from build123d import *

# Parameters (mm, degrees)
F0_R     = 10.925
F1_DEPTH = 8


with BuildPart() as f1:
    # F0 (on Front) → F1 (new body)
    with BuildSketch(Plane.XZ):
        Polygon((137.5925300597, 43.0939033628), (138.203267445, 43.0939033628), (132.6625055075, 50.7201079193), (132.6625055075, 44.6957654427), align=None)
        Polygon((132.6625055075, 66.4920412828), (138.3919956762, 68.353665488), (141.9330153387, 73.2274609315), (132.6625055075, 76.2396321698), align=None)
        with BuildLine():
            Line((152.4504447694, 74.5233945768), (153.3919956762, 73.2274609315))
            Line((153.3919956762, 73.2274609315), (162.6625055075, 76.2396321698))
            Line((162.6625055075, 76.2396321698), (162.6625055075, 93.0939033628))
            ThreePointArc((162.6625055075, 93.0939033628), (161.1980394134, 96.6294372687), (157.6625055075, 98.0939033628))
            Line((157.6625055075, 98.0939033628), (137.6625055075, 98.0939033628))
            ThreePointArc((137.6625055075, 98.0939033628), (134.1269716015, 96.6294372687), (132.6625055075, 93.0939033628))
            Line((132.6625055075, 93.0939033628), (132.6625055075, 76.2396321698))
            Line((132.6625055075, 76.2396321698), (141.9330153387, 73.2274609315))
            Line((141.9330153387, 73.2274609315), (142.8745662455, 74.5233945768))
            Line((142.8745662455, 74.5233945768), (146.8630398909, 71.6255988516))
            Line((146.8630398909, 71.6255988516), (147.6625055075, 71.3658367263))
            Line((147.6625055075, 71.3658367263), (148.461971124, 71.6255988516))
            Line((148.461971124, 71.6255988516), (152.4504447694, 74.5233945768))
        make_face()
        with Locations((147.6625055075, 85.5939033628)):
            Circle(F0_R, mode=Mode.SUBTRACT)
        Polygon((153.3919956762, 73.2274609315), (156.9330153387, 68.353665488), (162.6625055075, 66.4920412828), (162.6625055075, 76.2396321698), align=None)
        Polygon((147.9678742002, 71.2666164235), (156.9330153387, 68.353665488), (153.3919956762, 73.2274609315), (148.461971124, 71.6255988516), align=None)
        Polygon((138.5807239074, 43.0939033628), (156.7442871075, 43.0939033628), (162.3571368148, 60.3684785034), (147.6625055075, 71.0447530815), (132.9678742002, 60.3684785034), align=None)
        with Locations((147.6625055075, 55.5939033628)):
            Circle(F0_R, mode=Mode.SUBTRACT)
        Polygon((147.6625055075, 30.0743791122), (153.3919956762, 37.960345794), (147.6625055075, 39.8219699992), (141.9330153387, 37.960345794), align=None)
        with BuildLine():
            Line((137.7558134621, 16.4389872893), (147.6625055075, 30.0743791122))
            Line((147.6625055075, 30.0743791122), (141.9330153387, 37.960345794))
            Line((141.9330153387, 37.960345794), (140.4095539694, 37.4653431886))
            Line((140.4095539694, 37.4653431886), (138.8860926001, 42.1540751645))
            Line((138.8860926001, 42.1540751645), (138.3919956762, 42.8341412375))
            Line((138.3919956762, 42.8341412375), (137.5925300597, 43.0939033628))
            Line((137.5925300597, 43.0939033628), (132.6625055075, 43.0939033628))
            Line((132.6625055075, 43.0939033628), (132.6625055075, 44.6957654427))
            Line((132.6625055075, 44.6957654427), (123.3919956762, 47.707936681))
            Line((123.3919956762, 47.707936681), (113.4853036309, 34.0725448581))
            ThreePointArc((113.4853036309, 34.0725448581), (112.5919468998, 30.3514462714), (114.5914623413, 27.0885336247))
            Line((114.5914623413, 27.0885336247), (130.7718022288, 15.3328285789))
            ThreePointArc((130.7718022288, 15.3328285789), (134.4929008155, 14.4394718478), (137.7558134621, 16.4389872893))
        make_face()
        with Locations((130.0289479387, 31.3233935315)):
            Circle(F0_R, mode=Mode.SUBTRACT)
        with BuildLine():
            Line((162.6625055075, 44.6957654427), (162.6625055075, 43.0939033628))
            Line((162.6625055075, 43.0939033628), (157.7324809553, 43.0939033628))
            Line((157.7324809553, 43.0939033628), (156.9330153387, 42.8341412375))
            Line((156.9330153387, 42.8341412375), (156.4389184148, 42.1540751645))
            Line((156.4389184148, 42.1540751645), (154.9154570455, 37.4653431886))
            Line((154.9154570455, 37.4653431886), (153.3919956762, 37.960345794))
            Line((153.3919956762, 37.960345794), (147.6625055075, 30.0743791122))
            Line((147.6625055075, 30.0743791122), (157.5691975528, 16.4389872893))
            ThreePointArc((157.5691975528, 16.4389872893), (160.8321101995, 14.4394718478), (164.5532087862, 15.3328285789))
            Line((164.5532087861, 15.3328285789), (180.7335486736, 27.0885336247))
            ThreePointArc((180.7335486736, 27.0885336247), (182.7330641152, 30.3514462714), (181.8397073841, 34.0725448581))
            Line((181.8397073841, 34.0725448581), (171.9330153387, 47.707936681))
            Line((171.9330153387, 47.707936681), (162.6625055075, 44.6957654427))
        make_face()
        with Locations((165.2960630762, 31.3233935315)):
            Circle(F0_R, mode=Mode.SUBTRACT)
        with BuildLine():
            Line((166.20352517, 55.5939033628), (171.9330153387, 47.707936681))
            Line((171.9330153387, 47.707936681), (187.9623797842, 52.9161929074))
            ThreePointArc((187.9623797842, 52.9161929074), (190.8723274332, 55.4015229902), (191.1725773938, 59.2165604607))
            Line((191.1725773938, 59.2165604607), (184.9922375063, 78.2376907866))
            ThreePointArc((184.9922375063, 78.2376907866), (182.5069074235, 81.1476384357), (178.6918699529, 81.4478883962))
            Line((178.6918699529, 81.4478883962), (162.6625055075, 76.2396321698))
            Line((162.6625055075, 76.2396321698), (162.6625055075, 66.4920412828))
            Line((162.6625055075, 66.4920412828), (164.1859668768, 65.9970386775))
            Line((164.1859668768, 65.9970386775), (162.6625055075, 61.3083067016))
            Line((162.6625055075, 61.3083067016), (162.6625055075, 60.4676988062))
            Line((162.6625055075, 60.4676988062), (163.1566024313, 59.7876327333))
            Line((163.1566024313, 59.7876327333), (167.1450760767, 56.8898370081))
            Line((167.1450760767, 56.8898370081), (166.20352517, 55.5939033628))
        make_face()
        with Locations((176.1942009963, 64.864413194)):
            Circle(F0_R, mode=Mode.SUBTRACT)
        Polygon((162.6625055075, 50.7201079193), (162.6625055075, 44.6957654427), (171.9330153387, 47.707936681), (166.20352517, 55.5939033628), align=None)
        Polygon((162.6625055075, 60.1466151614), (162.6625055075, 50.7201079193), (166.20352517, 55.5939033628), (163.1566024313, 59.7876327333), align=None)
        Polygon((163.1566024313, 59.7876327333), (166.20352517, 55.5939033628), (167.1450760767, 56.8898370081), align=None)
        Polygon((156.7442871075, 43.0939033628), (157.1217435699, 43.0939033628), (162.6625055075, 50.7201079193), (162.6625055075, 60.1466151614), (162.3571368148, 60.3684785034), align=None)
        Polygon((157.1217435699, 43.0939033628), (157.7324809553, 43.0939033628), (162.6625055075, 44.6957654427), (162.6625055075, 50.7201079193), align=None)
        Polygon((157.7324809553, 43.0939033628), (162.6625055075, 43.0939033628), (162.6625055075, 44.6957654427), align=None)
        Polygon((154.9154570455, 37.4653431886), (156.4389184148, 42.1540751645), (153.3919956762, 37.960345794), align=None)
        Polygon((153.3919956762, 37.960345794), (156.4389184148, 42.1540751645), (156.627646646, 42.7349209346), (147.6625055075, 39.8219699992), align=None)
        Polygon((156.627646646, 42.7349209346), (156.7442871075, 43.0939033628), (138.5807239074, 43.0939033628), (138.6973643689, 42.7349209346), (147.6625055075, 39.8219699992), align=None)
        Polygon((141.9330153387, 37.960345794), (147.6625055075, 39.8219699992), (138.6973643689, 42.7349209346), (138.8860926001, 42.1540751645), align=None)
        Polygon((140.4095539694, 37.4653431886), (141.9330153387, 37.960345794), (138.8860926001, 42.1540751645), align=None)
        Polygon((138.203267445, 43.0939033628), (138.5807239074, 43.0939033628), (132.9678742002, 60.3684785034), (132.6625055075, 60.1466151614), (132.6625055075, 50.7201079193), align=None)
        Polygon((132.6625055075, 43.0939033628), (137.5925300597, 43.0939033628), (132.6625055075, 44.6957654427), align=None)
        Polygon((132.6625055075, 44.6957654427), (132.6625055075, 50.7201079193), (129.121485845, 55.5939033628), (123.3919956762, 47.707936681), align=None)
        Polygon((129.121485845, 55.5939033628), (132.6625055075, 50.7201079193), (132.6625055075, 60.1466151614), (132.1684085836, 59.7876327333), align=None)
        Polygon((128.1799349382, 56.8898370081), (129.121485845, 55.5939033628), (132.1684085836, 59.7876327333), align=None)
        Polygon((132.6625055075, 61.3083067016), (132.8512337387, 60.7274609315), (138.3919956762, 68.353665488), (132.6625055075, 66.4920412828), align=None)
        Polygon((131.1390441382, 65.9970386775), (132.6625055075, 61.3083067016), (132.6625055075, 66.4920412828), align=None)
        Polygon((132.8512337387, 60.7274609315), (132.9678742002, 60.3684785034), (147.6625055075, 71.0447530815), (147.3571368148, 71.2666164235), (138.3919956762, 68.353665488), align=None)
        Polygon((141.9330153387, 73.2274609315), (146.8630398909, 71.6255988516), (142.8745662455, 74.5233945768), align=None)
        Polygon((138.3919956762, 68.353665488), (147.3571368148, 71.2666164235), (146.8630398909, 71.6255988516), (141.9330153387, 73.2274609315), align=None)
        Polygon((147.6625055075, 71.0447530815), (162.3571368148, 60.3684785034), (162.4737772763, 60.7274609315), (156.9330153387, 68.353665488), (147.9678742002, 71.2666164235), align=None)
        Polygon((156.9330153387, 68.353665488), (162.4737772763, 60.7274609315), (162.6625055075, 61.3083067016), (162.6625055075, 66.4920412828), align=None)
        Polygon((162.6625055075, 66.4920412828), (162.6625055075, 61.3083067016), (164.1859668768, 65.9970386775), align=None)
        Polygon((148.461971124, 71.6255988516), (153.3919956762, 73.2274609315), (152.4504447694, 74.5233945768), align=None)
        with BuildLine():
            Line((123.3919956762, 47.707936681), (129.121485845, 55.5939033628))
            Line((129.121485845, 55.5939033628), (128.1799349382, 56.8898370081))
            Line((128.1799349382, 56.8898370081), (132.1684085836, 59.7876327333))
            Line((132.1684085836, 59.7876327333), (132.6625055075, 60.4676988062))
            Line((132.6625055075, 60.4676988062), (132.6625055075, 61.3083067016))
            Line((132.6625055075, 61.3083067016), (131.1390441382, 65.9970386775))
            Line((131.1390441382, 65.9970386775), (132.6625055075, 66.4920412828))
            Line((132.6625055075, 66.4920412828), (132.6625055075, 76.2396321698))
            Line((132.6625055075, 76.2396321698), (116.633141062, 81.4478883962))
            ThreePointArc((116.633141062, 81.4478883962), (112.8181035915, 81.1476384357), (110.3327735087, 78.2376907866))
            Line((110.3327735087, 78.2376907866), (104.1524336212, 59.2165604607))
            ThreePointArc((104.1524336212, 59.2165604607), (104.4526835817, 55.4015229902), (107.3626312308, 52.9161929074))
            Line((107.3626312308, 52.9161929074), (123.3919956762, 47.707936681))
        make_face()
        with Locations((119.1308100186, 64.864413194)):
            Circle(F0_R, mode=Mode.SUBTRACT)
    extrude(amount=F1_DEPTH)


solid = f1.part
Can you work these out from the model? Positions are in its coordinate system, mm. A direction names the side the tool comes from. Coordinates: 2 decimals unless noted, no trailing zeros. Order: outer loops, then holes, each group sorted by start corner. A loop starts at its lowest first (then second) coordinate and runs counter-clockwise, first axis right, second up. Notation, with made-up numbers: M 75.25,12.5 L 110.25,12.5 A16 cw 110.25,26.5 Z; hole C 2,71 d5. An arc over 180 degrees is marked long. Write item = value, one per line.
(1) Suppose I cut it at C-C on z = 38. Please give me the cut outline in (x, y), plus the area to 3 significant figures.
Results are:
outline = M 116.34,-8 L 121.38,-8 L 121.38,0 L 116.34,0 Z; M 138.68,-8 L 156.65,-8 L 156.65,0 L 138.68,0 Z; M 173.94,-8 L 178.99,-8 L 178.99,0 L 173.94,0 Z
area = 224 mm2
(2) For pin 1 Ø0.8 at (x, y) = (157.5, -3.5) entering from -Z; pin 2 Ø4 at (y, z) = (-3.5, 82) entering from -X; pin 3 Ø3 at (x, y) = (166.5, -1.5) entering from +Z, each with a flat end and sliding along its axis, tell me the tip position at first contact or that it passes through.
Results are:
pin_1 = 16.03
pin_2 = 111.34
pin_3 = 77.97
(3) I need wall thicknesses on line 1 along X through (y, z) = (-1.25, 90); line 2 along X through (y, z) = (-5, 29); line 3 along X through (y, z) = (-4.75, 55.5). Which ranges of each line are inside material? Lowest first, please. Write a range as [from, to].
Results are:
line_1 = [132.66, 137.67], [157.66, 162.66]
line_2 = [113.01, 119.35], [140.7, 146.88], [148.44, 154.62], [175.97, 182.32]
line_3 = [104.4, 113.5], [124.76, 136.74], [158.59, 170.57], [181.82, 190.92]
(4) Suppose I cut it at A-A on z = 51. Please give me the cut outline in (x, y).
Results are:
outline = M 113.26,-8 L 137.75,-8 L 137.75,0 L 113.26,0 Z; M 157.57,-8 L 182.06,-8 L 182.06,0 L 157.57,0 Z
(5) Suppose I cut it at D-D on y = -2.5. State how many separate pieces and enclosed holes the cut face has, plus the area to 3 significant figures.
Results are:
separate_pieces = 1
enclosed_holes = 11
area = 2,520 mm2
(6) Suppose I cut it at B-B on x = 134.5. Please give me the cut outline in (y, z).
Results are:
outline = M -8,14.44 L 0,14.44 L 0,21.36 L -8,21.36 Z; M -8,41.29 L 0,41.29 L 0,96.97 L -8,96.97 Z
(7) For faces 1 (the face through (179.835, -3.944, 50.276)), 2 (the face through (170.79, -3.94, 78.88)), 3 (the face through (152.55, -3.94, 23.35)), 4 (the face through (136.748, -3.944, 56.074)), which set-ups out of +Z, -Z, +X, -X, +Y, -Y let a thin tool reach every point of the face, with its end or its side?
Results are:
face_1 = +X, +Y, -Y
face_2 = +Z, +Y, -Y
face_3 = -Z, +Y, -Y
face_4 = +Y, -Y
(8) If we mould it in two halves opening along X, with no side actions, what happens to faces 5 (the face through (182.724, -3.944, 30.297)), 6 (the face through (116.76, -3.94, 54.2)), 7 (the face through (148, -4, 98.094)), 8 (the face through (132.663, -4, 85))? For each: pulls with the +X half, pulls with the -X half, needs draft (parallel to the pull), parting line crosses it, or undercut.
Results are:
face_5 = pulls with the +X half
face_6 = undercut
face_7 = needs draft
face_8 = undercut
